Part model, mm, in its own coordinate system. A direction names the side the tool comes from. Round coordinates to 2 decimals unless told otherwise and drop trailing zeros. Loops run counter-clockwise (first coordinate to the right, second up) from the corner with the lowest first, then second, coordinate; pieces in that order, holes last.
from build123d import *

# Parameters (mm, degrees)
SKETCH1_R                    = 25
BOSS_EXTRUDE1_DEPTH          = 15
CUT_EXTRUDE1_DEPTH           = 30
CUT_EXTRUDE_THIN3_DEPTH      = 26
CUT_EXTRUDE_THIN3_DEPTH_BACK = 26


with BuildPart() as part:
    # Sketch1 → Boss-Extrude1 (new body, symmetric)
    with BuildSketch(Plane.XY):
        Circle(SKETCH1_R)
    extrude(amount=BOSS_EXTRUDE1_DEPTH, both=True)

    # Sketch2 → Cut-Extrude1 (cut)
    with BuildSketch(Plane.XY.offset(15)):
        Polygon((-128.64988892, 86.933618644), (-20.714125317, 13.997321614), (0, 0), (14.35317498, 20.469156504), (89.143728668, 127.128453183), (41.85899915, 383.338297472), (-175.934618438, 343.143462933), align=None)
    extrude(amount=-CUT_EXTRUDE1_DEPTH, mode=Mode.SUBTRACT)

    # Sketch4 → Cut-Extrude-Thin3 (cut, two sides)
    with BuildSketch(Plane(origin=(0, 0, 0), x_dir=(0, 0, -1), z_dir=(1, 0, 0))) as cut_extrude_thin3_sk:
        Polygon((-8.132669534, -9.679737666), (7.600765094, -4.847746507), (7.30718246, -3.891812808), (-8.426252168, -8.723803967), align=None)
    extrude(amount=CUT_EXTRUDE_THIN3_DEPTH, mode=Mode.SUBTRACT)
    extrude(cut_extrude_thin3_sk.sketch, amount=-CUT_EXTRUDE_THIN3_DEPTH_BACK, mode=Mode.SUBTRACT)


solid = part.part
1) Slice it at D-D, the plane x = -15.5. Give the cut face in (y, z).
Values:
outline: (-19.62, -15) - (10.47, -15) - (10.47, 15) - (-19.62, 15) - close; hole (-9.68, 8.13) - (-4.85, -7.6) - (-3.89, -7.31) - (-8.72, 8.43) - close
2) Slice it at C-C, the plane x = 12. Give the cut face in (y, z).
Values:
outline: (-21.93, -15) - (17.11, -15) - (17.11, 15) - (-21.93, 15) - close; hole (-9.68, 8.13) - (-4.85, -7.6) - (-3.89, -7.31) - (-8.72, 8.43) - close
3) Mould opens along Z. For faces 4 (the face through (0, -7, -15)), 5 (the face through (-10.502, 7.097, 0.21)), 6 (the face through (0.34, -7.3, 0.38)) say: released by +Z, released by -Z, zero draft, split by the parting line, or undercut.
Values:
face 4: released by -Z
face 5: zero draft
face 6: undercut
4) Drop flat-ended pins along their axis: pin 1 Ø10 at (x, z) = (19.5, -11) entering from +Y; pin 2 Ø1 at (x, z) = (-19, 4.5) entering from +Y; pin 3 Ø6 at (x, z) = (13, 5.5) entering from +Y. Give the stop position or say it passes through.
Values:
pin 1: stops at y = 20.37
pin 2: stops at y = 13.18
pin 3: stops at y = 20.47
5) Slice it at B-B, the plane y = 7.5. Give the cut face in (x, z), then the cut area to 3 significant figures.
Values:
outline: (-23.85, -15) - (-11.1, -15) - (-11.1, 15) - (-23.85, 15) - close; (5.26, -15) - (23.85, -15) - (23.85, 15) - (5.26, 15) - close
area: 940 mm2
6) Slice it at A-A, the plane z = -1.25. Give the cut face in (x, y), then the cut area to 3 significant figures.
Values:
outline: (-24.33, -5.75) - (24.33, -5.75) arc R25 ccw to (14.35, 20.47) - (0, 0) - (-20.71, 14) arc R25 ccw to start; (-24.06, -6.8) arc R25 ccw to (24.06, -6.8) - close
area: 1,420 mm2
7) Wall check: line 1 along X through (y, z) = (1.5, 4.75); line 2 along X through (y, z) = (11, 4); line 3 along Y through (x, z) = (-6.5, 7.5). Give the ranges that are in metal, low to high.
Values:
line 1: x = -24.95 to -2.22, 1.05 to 24.95
line 2: x = -22.45 to -16.28, 7.71 to 22.45
line 3: y = -24.14 to -9.49, -8.44 to 4.39
8) Tool access for faces 1 (the face through (7.076, 10.091, 0.21)), 2 (the face through (0.346, -6.274, 0.449)), 3 (the face through (0, -7, 15)): list every direction of +Z, -Z, +X, -X, +Y, -Y with a clear straight run to the whole face (end or side of a thin tool).
Values:
face 1: +Z, -Z, +Y
face 2: +X, -X
face 3: +Z, +X, -X, +Y, -Y
